from build123d import *

# Parameters (mm, degrees)
SKETCH1_W               = 9
SKETCH1_H               = 7
BOSS_EXTRUDE1_DEPTH     = 6
SKETCH2_W               = 3
SKETCH2_H               = 2
CUT_EXTRUDE1_DEPTH      = 12.368817001
SKETCH3_W               = 3
SKETCH3_H               = 2
CUT_EXTRUDE2_DEPTH      = 8
CHAMFER1_SIZE           = 1
SKETCH4_W               = 1
SKETCH4_H               = 2
CUT_EXTRUDE3_DEPTH      = 9.276472679
SKETCH5_W               = 3
SKETCH5_H               = 2
CUT_EXTRUDE4_DEPTH      = 2
CHAMFER2_SIZE           = 2
CUT_EXTRUDE5_DEPTH      = 2
CUT_EXTRUDE5_DEPTH_BACK = 1
CUT_EXTRUDE6_DEPTH      = 5.094054233
CUT_EXTRUDE7_DEPTH      = 5.094054233


with BuildPart() as part:
    # Sketch1 → Boss-Extrude1 (new body)
    with BuildSketch(Plane(origin=(0, 0, 0), x_dir=(1, 0, 0), z_dir=(0, 1, 0))):
        Rectangle(SKETCH1_W, SKETCH1_H)
    extrude(amount=BOSS_EXTRUDE1_DEPTH)

    # Sketch2 → Cut-Extrude1 (cut, through all)
    with BuildSketch(Plane.ZY.offset(4.5)):
        with Locations((1, 1)):
            Rectangle(SKETCH2_W, SKETCH2_H)
    extrude(amount=-CUT_EXTRUDE1_DEPTH, mode=Mode.SUBTRACT)

    # Sketch3 → Cut-Extrude2 (cut)
    with BuildSketch(Plane.ZY.offset(4.5)):
        with Locations((2, 5)):
            Rectangle(SKETCH3_W, SKETCH3_H)
    extrude(amount=-CUT_EXTRUDE2_DEPTH, mode=Mode.SUBTRACT)

    # Chamfer1
    chamfer1_edges = [part.edges().sort_by_distance(p)[0] for p in [
        (4, 6, 3.5),
    ]]
    chamfer(chamfer1_edges, length=CHAMFER1_SIZE)

    # Sketch4 → Cut-Extrude3 (cut, through all)
    with BuildSketch(Plane(origin=(0, 6, 0), x_dir=(1, 0, 0), z_dir=(0, 1, 0))):
        with Locations((4, 2.5)):
            Rectangle(SKETCH4_W, SKETCH4_H)
    extrude(amount=-CUT_EXTRUDE3_DEPTH, mode=Mode.SUBTRACT)

    # Sketch5 → Cut-Extrude4 (cut)
    with BuildSketch(Plane(origin=(0, 6, 0), x_dir=(1, 0, 0), z_dir=(0, 1, 0))):
        with Locations((-3, 0.5)):
            Rectangle(SKETCH5_W, SKETCH5_H)
    extrude(amount=-CUT_EXTRUDE4_DEPTH, mode=Mode.SUBTRACT)

    # Chamfer2
    chamfer2_edges = [part.edges().sort_by_distance(p)[0] for p in [
        (-4.5, 6, -2.5),
    ]]
    chamfer(chamfer2_edges, length=CHAMFER2_SIZE)

    # Sketch6 → Cut-Extrude5 (cut, two sides)
    with BuildSketch(Plane.XY.offset(-1.5)) as cut_extrude5_sk:
        Polygon((-4.5, 4), (-2.5, 6), (-0.5, 6), (-1.5, 4), align=None)
    extrude(amount=CUT_EXTRUDE5_DEPTH, mode=Mode.SUBTRACT)
    extrude(cut_extrude5_sk.sketch, amount=-CUT_EXTRUDE5_DEPTH_BACK, mode=Mode.SUBTRACT)

    # Sketch7 → Cut-Extrude6 (cut)
    with BuildSketch(Plane(origin=(0, 4, 0), x_dir=(1, 0, 0), z_dir=(0, 1, 0))):
        Polygon((-4.5, 1.5), (-3.5, 1.5), (-3.5, 0.5), (-2.5, 0.5), (-2.5, -3.5), (-4.5, -3.5), align=None)
    extrude(amount=-CUT_EXTRUDE6_DEPTH, mode=Mode.SUBTRACT)

    # 3DSketch1 → Cut-Extrude7 (cut, along a direction that is not the sketch's normal)
    with BuildSketch(Plane(origin=(2.5, 4, 3.5), x_dir=(-0.7453559924999292, -0.29814239699997236, -0.5962847939999446), z_dir=(0.6666666666666674, -0.33333333333333376, -0.6666666666666657))):
        Polygon((0, 0), (2.683281573, -3.577708764), (4.024922359, -3.130495168), (2.683281573, -1.341640786), (6.708203932, 0), (4.024922359, 3.577708764), (2.683281573, 3.130495168), (4.024922359, 1.341640786), align=None)
    extrude(amount=-CUT_EXTRUDE7_DEPTH, dir=(1, 0, 0), mode=Mode.SUBTRACT)


solid = part.part
Input: part model. Units: mm. Frame: model coordinates. A direction names the side the tool comes from. Coordinates: 2 decimals unless noted, no trailing zeros. Order: outer loops, then holes, each group sorted by start corner. A loop starts at its lowest first (then second) coordinate and runs counter-clockwise, first axis right, second up.
1. Ray query, line 1 along Z through (x, y) = (4, 0.5); line 2 along Z through (x, y) = (1.5, 0.5); line 3 along Z through (x, y) = (-1.5, 4.5). Return the intervals inside material, ascending.
Checked values:
line 1: z = -1.5 to -0.5, 2.5 to 3.5
line 2: z = -3.5 to -0.5, 2.5 to 3.5
line 3: z = -3.5 to -2.5
2. Access query for faces 1 (the flat face through (-3.5, 2, -1)), 2 (the flat face through (4, 3, -1.5)), 3 (the flat face through (-3, 4, -2)), 4 (the flat face through (2, 0, 3)), 5 (the flat face through (2, 1, 2.5)). Directions: +Z, -Z, +X, -X, +Y, -Y. A direction counts if a zero-diameter tool reaches every point of the face in a straight line with its end or side. Return the directions, or none.
Checked values:
face 1: +Z, -X, +Y, -Y
face 2: -Z, +X, +Y, -Y
face 3: +Z, -X, +Y
face 4: +Z, -Z, +X, -X, -Y
face 5: +X, -X, -Y
3. Contact query for flat-ended pins moving along their axis: P1, Ø2.5, axis at x = 1.5, z = 2, coming from the +Y side; P2, Ø4, axis at x = -3.5, z = -1, coming from the +Y side; P3, Ø0.5, axis at x = -4, y = 1.5, coming from the +Z side; P4, Ø1.5, axis at x = 1.5, z = 0.5, coming from the -Y side. Output: stop coordinate, or through.
Checked values:
P1: stops at y = 4
P2: stops at y = 6
P3: stops at z = -1.5
P4: stops at y = 2
4. Cut plane A-A, the plane y = 1. Return loops of the section in (x, z), plus the area to 3 significant figures.
Checked values:
outline: (-4.5, -3.5) - (3.5, -3.5) - (3.5, -1.5) - (4.5, -1.5) - (4.5, -0.5) - (-3.5, -0.5) - (-3.5, -1.5) - (-4.5, -1.5) - close; (0, 2.5) - (4.5, 2.5) - (4.5, 3.5) - (1, 3.5) - close
area: 28.0 mm2
5. Cut plane D-D, the plane z = 1. Return loops of the section in (x, y).
Checked values:
outline: (-1, 2) - (4.5, 2) - (4.5, 6) - (3.5, 6) - (3.5, 4) - (0, 4) - close
6. Cut plane B-B, the plane x = 1. Return loops of the section in (y, z).
Checked values:
outline: (0, -3.5) - (6, -3.5) - (6, 0.5) - (4, 0.5) - (4, 2) - (1, 3.5) - (0, 3.5) - (0, 2.5) - (2, 2.5) - (2, -0.5) - (0, -0.5) - close
7. Cut plane C-C, the plane y = 4.5. Return loops of the section in (x, z), plus the area to 4 significant figures.
Checked values:
outline: (-4, -3.5) - (3.5, -3.5) - (3.5, -1.5) - (4.5, -1.5) - (4.5, 3.5) - (3.5, 3.5) - (3.5, 0.5) - (-0.25, 0.5) - (-1.25, -0.5) - (-1.25, -2.5) - (-4, -2.5) - close
area: 26.25 mm2
